```python
from build123d import *

# Parameters (mm, degrees)
F1_DEPTH = 25


with BuildPart() as f1:
    # F0 (on Top) → F1 (new body)
    with BuildSketch(Plane.XY):
        Polygon((-83.662644, 46.76469), (-46.76469, -83.662644), (83.662644, -46.76469), (46.76469, 83.662644), align=None)
    extrude(amount=F1_DEPTH)

    # F1_face (on face) → F4 section 0
    with BuildSketch(Plane.XY.offset(25), mode=Mode.PRIVATE) as f4_s0:
        Polygon((83.662644, -46.76469), (46.76469, 83.662644), (-83.662644, 46.76469), (-46.76469, -83.662644), align=None)
    loft([Vertex(-2.560169, 2.400158, 100), f4_s0.sketch])


solid = f1.part
```
For this review, take the finished solid that the model builds, in its own axes (mm). Coordinates: 2 decimals unless noted, no trailing zeros. Loops run counter-clockwise (first coordinate to the right, second up) from the corner with the lowest first, then second, coordinate; pieces in that order, holes last. Notation, with made-up numbers: (68, 63) -> (111, 63) arc R32 ccw to (111, 94) -> close; hole circle Ø9 at (-29, 39.5). An arc over 180 degrees is marked (long way). Return JSON: item names as keys, results as strings. Group by question number.
(1) Consider section B-B, the plane x = -27. Give the boundary of the cut face in (y, z).
(2) Consider section A-A, the plane z = 13.5. Give the boundary of the cut face in (x, y).
(3) Consider section D-D, the plane x = -56. Give the boundary of the cut face in (y, z), plus the area to 3 significant figures.
(4) For pin 1 Ø10 at (x, y) = (-39, 36.5) entering from +Z; pin 2 Ø6 at (x, y) = (46.5, -34) entering from +Z; pin 3 Ø1.5 at (x, y) = (36.5, 14) entering from +Z, all flat-tipped, find the tip position at first contact; note any pin that passes through.
(5) Consider section C-C, the plane y = -2. Give the boundary of the cut face in (x, z), plus the area to 3 significant figures.
(6) To check wall thickness, follow L1, parallel to Y at x = 37.5, z = 17; L2, parallel to Z at x = 64, y = 4; L3, parallel to Y at x = -10.5, z = 47. State the ranges of each line that lie inside material, in increasing order.
Results below:
{
 "1": {"outline": "(-78.07, 0) -> (62.79, 0) -> (62.79, 25) -> (15.77, 77.4) -> (-45.18, 58.53) -> (-78.07, 25) -> close"},
 "2": {"outline": "(-83.66, 46.76) -> (-46.76, -83.66) -> (83.66, -46.76) -> (46.76, 83.66) -> close"},
 "3": {"outline": "(-51.02, 0) -> (54.59, 0) -> (54.59, 25) -> (31.63, 50.58) -> (-51.02, 25) -> close", "area": "3,990 mm2"},
 "4": {"pin 1": "stops at z = 56.31", "pin 2": "stops at z = 51.91", "pin 3": "stops at z = 56.89"},
 "5": {"outline": "(-69.87, 0) -> (71, 0) -> (71, 25) -> (5.16, 93.29) -> (-4.82, 96.17) -> (-69.87, 25) -> close", "area": "8,780 mm2"},
 "6": {"L1": "y = -59.82 to 81.04", "L2": "z = 0 to 30.5", "L3": "y = -51.83 to 47.72"}
}
